from build123d import *

# Parameters (mm, degrees)
F0_R     = 10
F1_DEPTH = 10
F2_R     = 15
F2_R_2   = 10
F3_DEPTH = 14
F4_R     = 3
F5_DEPTH = 5
F6_R     = 4.5
F7_DEPTH = 5
F8_R     = 12
F9_DEPTH = 5
F10_R    = 1


with BuildPart() as f1:
    # F0 (on Top) → F1 (new body)
    with BuildSketch(Plane.XY):
        with BuildLine():
            ThreePointArc((42, 0), (40.486347, 4.347413), (36.6, 6.81469))
            ThreePointArc((36.6, 6.81469), (28, 0), (36.6, -6.81469))
            ThreePointArc((36.6, -6.81469), (40.486347, -4.347413), (42, 0))
        make_face()
        with BuildLine():
            ThreePointArc((-28, 0), (-30.652587, 5.486347), (-36.6, 6.81469))
            ThreePointArc((-36.6, 6.81469), (-42, 0), (-36.6, -6.81469))
            ThreePointArc((-36.6, -6.81469), (-30.652587, -5.486347), (-28, 0))
        make_face()
        with BuildLine():
            ThreePointArc((3.428571, 14.602907), (11.756457, 9.315885), (15, 0))
            ThreePointArc((15, 0), (11.756457, -9.315885), (3.428571, -14.602907))
            Line((3.428571, -14.602907), (36.6, -6.81469))
            ThreePointArc((36.6, -6.81469), (28, 0), (36.6, 6.81469))
            Line((36.6, 6.81469), (3.428571, 14.602907))
        make_face()
        with BuildLine():
            ThreePointArc((3.428571, -14.602907), (11.756457, -9.315885), (15, 0))
            ThreePointArc((15, 0), (11.756457, 9.315885), (3.428571, 14.602907))
            ThreePointArc((3.428571, 14.602907), (0, 15), (-3.428571, 14.602907))
            ThreePointArc((-3.428571, 14.602907), (-15, 0), (-3.428571, -14.602907))
            ThreePointArc((-3.428571, -14.602907), (0, -15), (3.428571, -14.602907))
        make_face()
        Circle(F0_R, mode=Mode.SUBTRACT)
        with BuildLine():
            ThreePointArc((-3.428571, -14.602907), (-15, 0), (-3.428571, 14.602907))
            Line((-3.428571, 14.602907), (-36.6, 6.81469))
            ThreePointArc((-36.6, 6.81469), (-30.652587, 5.486347), (-28, 0))
            ThreePointArc((-28, 0), (-30.652587, -5.486347), (-36.6, -6.81469))
            Line((-36.6, -6.81469), (-3.428571, -14.602907))
        make_face()
    extrude(amount=F1_DEPTH)

    # F2 (on face) → F3 (join)
    with BuildSketch(Plane.XY.offset(10)):
        Circle(F2_R)
        Circle(F2_R_2, mode=Mode.SUBTRACT)
        with BuildLine():
            ThreePointArc((3.428571, -14.602907), (11.756457, -9.315885), (15, 0))
            ThreePointArc((15, 0), (11.756457, 9.315885), (3.428571, 14.602907))
            ThreePointArc((3.428571, 14.602907), (0, 15), (-3.428571, 14.602907))
            ThreePointArc((-3.428571, 14.602907), (-15, 0), (-3.428571, -14.602907))
            ThreePointArc((-3.428571, -14.602907), (0, -15), (3.428571, -14.602907))
        make_face()
        Circle(F2_R_2, mode=Mode.SUBTRACT)
    extrude(amount=F3_DEPTH)

    # F4 (on Top) → F5 (cut)
    with BuildSketch(Plane.XY):
        with Locations((35, 0)):
            Circle(F4_R)
        with Locations((-35, 0)):
            Circle(F4_R)
    extrude(amount=F5_DEPTH, mode=Mode.SUBTRACT)

    # F6 (on face) → F7 (cut)
    with BuildSketch(Plane.XY.offset(10)):
        with Locations((35, 0)):
            Circle(F6_R)
        with Locations((-35, 0)):
            Circle(F6_R)
    extrude(amount=-F7_DEPTH, mode=Mode.SUBTRACT)

    # F8 (on face) → F9 (cut)
    with BuildSketch(Plane.XY.offset(24)):
        Circle(F8_R)
    extrude(amount=-F9_DEPTH, mode=Mode.SUBTRACT)

    # F10
    f10_edges = [f1.edges().sort_by_distance(p)[0] for p in [
        (-15, 0, 24),
    ]]
    fillet(f10_edges, radius=F10_R)


solid = f1.part
Work out the finished part from the listing and answer in its coordinate system (mm). A direction names the side the tool comes from. Give positions to 0.01 mm unless a question says otherwise; leave off trailing zeros. Loops run counter-clockwise (first coordinate to the right, second up) from the corner with the lowest first, then second, coordinate; pieces in that order, holes last. Notation, with made-up numbers: (58.25, 26) - (81.25, 26) arc R18 cw to (81.25, 59) - close; hole circle Ø1 at (-3, 74.5). An arc over 180 degrees is marked (long way). Answer in a Markdown table with one row per item. Add a question column.
Q1. Determine the mould class of faces 4 (the flat face through (-19.782, 10.763, 4.93)), 5 (the flat face through (-20.246, -10.654, 4.93)), 6 (the flat face through (-34, -3, 5)) for opening direction Y: released by +Y, released by -Y, zero draft, split by the parting line, or undercut.
Q2. The part is cut by section B-B (x = 0). Determine the outline of the cut face in (y, z), and give its area (3 significant figures).
Q3. Consider line 1 along X through (y, z) = (-0.5, 13); line 2 along X through (y, z) = (-3, 8); line 3 along Y through (x, z) = (35, 1.75). Determine where each line is inside the solid, lowest interval first.
Q4. A tool of negligible diameter and unlimited length cuts with its end or side. For faces 1 (the flat face through (36, -3, 5)), 2 (the cylindrical face through (15, 0, 16)), 3 (the cylindrical face through (-2.17, -9.76, 9.37)), from which of +Z, -Z, +X, -X, +Y, -Y can it reach the whole face along a straight path? Write none if from no direction.
Q5. The part is cut by section D-D (z = 2.25). Determine the outline of the cut face in (x, y), and give its area (3 significant figures).
Q6. Each of these flat-tipped pins is pushed along its axis until it touches: P1, Ø7, axis at x = -34.5, y = -2, coming from the +Z side; P2, Ø1, axis at x = 33, y = 2.5, coming from the +Z side; P3, Ø14.5, axis at x = 0, y = 0, coming from the +Z side; P4, Ø6, axis at x = -13.5, z = 6, coming from the -Y side. Where does it stop, or does it pass through?
Q7. The part is cut by section A-A (z = 9). Determine the outline of the cut face in (x, y), and give its area (3 significant figures).
Q8. The part is cut by section C-C (z = 20). Determine the outline of the cut face in (x, y).
Solution:
| question | item | result |
|---|---|---|
| 1 | face 4 | released by +Y |
| 1 | face 5 | released by -Y |
| 1 | face 6 | undercut |
| 2 | outline | (-15, 0) - (-10, 0) - (-10, 19) - (-12, 19) - (-12, 24) - (-14, 24) arc R1 ccw to (-15, 23) - close; (10, 0) - (15, 0) - (15, 23) arc R1 ccw to (14, 24) - (12, 24) - (12, 19) - (10, 19) - close |
| 2 | area | 220 mm² |
| 3 | line 1 | x = -14.99 to -9.99, 9.99 to 14.99 |
| 3 | line 2 | x = -41.32 to -38.35, -31.65 to -9.54, 9.54 to 31.65, 38.35 to 41.32 |
| 3 | line 3 | y = -7.19 to -3, 3 to 7.19 |
| 4 | face 1 | +Z |
| 4 | face 2 | +Z, +X |
| 4 | face 3 | +Z, -Z |
| 5 | outline | (-36.6, -6.81) - (-3.43, -14.6) arc R15 ccw to (3.43, -14.6) - (36.6, -6.81) arc R7 ccw to (42, 0) arc R7 ccw to (36.6, 6.81) - (3.43, 14.6) arc R15 ccw to (-3.43, 14.6) - (-36.6, 6.81) arc R7 ccw to start; hole circle Ø6 at (-35, 0); hole circle Ø20 at (0, 0); hole circle Ø6 at (35, 0) |
| 5 | area | 1,360 mm² |
| 6 | P1 | stops at z = 10 |
| 6 | P2 | stops at z = 5 |
| 6 | P3 | passes through |
| 6 | P4 | stops at y = -12.94 |
| 7 | outline | (-36.6, -6.81) - (-3.43, -14.6) arc R15 ccw to (3.43, -14.6) - (36.6, -6.81) arc R7 ccw to (42, 0) arc R7 ccw to (36.6, 6.81) - (3.43, 14.6) arc R15 ccw to (-3.43, 14.6) - (-36.6, 6.81) arc R7 ccw to start; hole circle Ø9 at (-35, 0); hole circle Ø20 at (0, 0); hole circle Ø9 at (35, 0) |
| 7 | area | 1,290 mm² |
| 8 | outline | (-3.43, -14.6) arc R15 ccw to (3.43, -14.6) arc R15 ccw to (3.43, 14.6) arc R15 ccw to (-3.43, 14.6) arc R15 ccw to start; hole circle Ø24 at (0, 0) |
